from build123d import *

# Parameters (mm, degrees)
CROQUIS1_R              = 12.5
SALIENTE_EXTRUIR1_DEPTH = 2.5
SALIENTE_EXTRUIR2_DEPTH = 10
CROQUIS3_R              = 5
CORTAR_EXTRUIR1_DEPTH   = 22.650635095


with BuildPart() as part:
    # Croquis1 → Saliente-Extruir1 (new body)
    with BuildSketch(Plane(origin=(0, 0, 0), x_dir=(1, 0, 0), z_dir=(0, 1, 0))):
        with Locations(Location((0, 0, 0), (0, 0, 270))):
            Circle(CROQUIS1_R)
    extrude(amount=SALIENTE_EXTRUIR1_DEPTH)

    # Croquis2 → Saliente-Extruir2 (add)
    with BuildSketch(Plane(origin=(0, 2.5, 0), x_dir=(1, 0, 0), z_dir=(0, 1, 0))):
        with BuildLine():
            Line((-7.5, 6.614378278), (-7.5, -6.614378278))
            ThreePointArc((-7.5, -6.614378278), (0, -10), (7.5, -6.614378278))
            Line((7.5, -6.614378278), (7.5, 6.614378278))
            ThreePointArc((7.5, 6.614378278), (0, 10), (-7.5, 6.614378278))
        make_face()
    extrude(amount=SALIENTE_EXTRUIR2_DEPTH)

    # Croquis3 → Cortar-Extruir1 (cut, through all)
    with BuildSketch(Plane(origin=(0, 12.5, 0), x_dir=(1, 0, 0), z_dir=(0, 1, 0))):
        with Locations(Location((0, 0, 0), (0, 0, 270))):
            Circle(CROQUIS3_R)
    extrude(amount=-CORTAR_EXTRUIR1_DEPTH, mode=Mode.SUBTRACT)


solid = part.part
Design review of the part built by this model. Coordinates are the model's own, in mm. A direction names the side the tool comes from. Coordinates: 2 decimals unless noted, no trailing zeros. Loops run counter-clockwise (first coordinate to the right, second up) from the corner with the lowest first, then second, coordinate; pieces in that order, holes last. Notation, with made-up numbers: M -10,-36 L -2,-36 A5 ccw -2,-28 Z; hole C 47,-25 d2. An arc over 180 degrees is marked long. Answer as CSV lines item,"result".
Item 1: Add section D-D on x = 6.5. State the section outline as (y, z) points, plus the area to 3 significant figures.
Answer list:
outline,"M 0,-10.68 L 2.5,-10.68 L 2.5,-7.6 L 12.5,-7.6 L 12.5,7.6 L 2.5,7.6 L 2.5,10.68 L 0,10.68 Z"
area,"205 mm²"
Item 2: Add section A-A on z = 0. State the section outline as (x, y) points, plus the area to 3 significant figures.
Answer list:
outline,"M -12.5,0 L -5,0 L -5,12.5 L -7.5,12.5 L -7.5,2.5 L -12.5,2.5 Z; M 5,0 L 12.5,0 L 12.5,2.5 L 7.5,2.5 L 7.5,12.5 L 5,12.5 Z"
area,"87.5 mm²"
Item 3: For probe 1 along X at (y, z) = (9, 0); probe 2 along Z at (x, y) = (0.25, 7.25); probe 3 along X at (y, z) = (10, 5.75), list the stretches that pass through material, from the lowest coordinate up.
Answer list:
probe 1,"-7.5 to -5, 5 to 7.5"
probe 2,"-10 to -4.99, 4.99 to 10"
probe 3,"-7.5 to 7.5"
Item 4: For P1, Ø5, axis at y = 7.5, z = 0, coming from the +X side; P2, Ø2, axis at x = -8, y = 10, coming from the -Z side; P3, Ø6, axis at x = 7.5, y = 3.5, coming from the +Z side, all flat-tipped, find the tip position at first contact; note any pin that passes through.
Answer list:
P1,"x = 7.5"
P2,"z = -7.14"
P3,"z = 11.59"
Item 5: Add section C-C on y = 10.25. State the section outline as (x, z) points, plus the area to 3 significant figures.
Answer list:
outline,"M -7.5,-6.61 A10 ccw 7.5,-6.61 L 7.5,6.61 A10 ccw -7.5,6.61 Z; hole C 0,0 d10"
area,"190 mm²"
Item 6: Add section B-B on x = 0. State the section outline as (y, z) points.
Answer list:
outline,"M 0,-12.5 L 2.5,-12.5 L 2.5,-10 L 12.5,-10 L 12.5,-5 L 0,-5 Z; M 0,5 L 12.5,5 L 12.5,10 L 2.5,10 L 2.5,12.5 L 0,12.5 Z"
Item 7: Machinability: for faces 1 (the face through (-7.5, 7, 0)), 2 (the face through (-8, 2.5, 0)), 3 (the face through (0, 7, 10)), 4 (the face through (7.5, 7, 0)), 5 (the face through (0, 7, -10)), which of the approach directions +Z, -Z, +X, -X, +Y, -Y give a long, thin tool a straight path to every point of the face, cutting with its end or side? Answer none if there is none.
Answer list:
face 1,"+Z, -Z, -X, +Y"
face 2,"+Y"
face 3,"+Z, +Y"
face 4,"+Z, -Z, +X, +Y"
face 5,"-Z, +Y"
